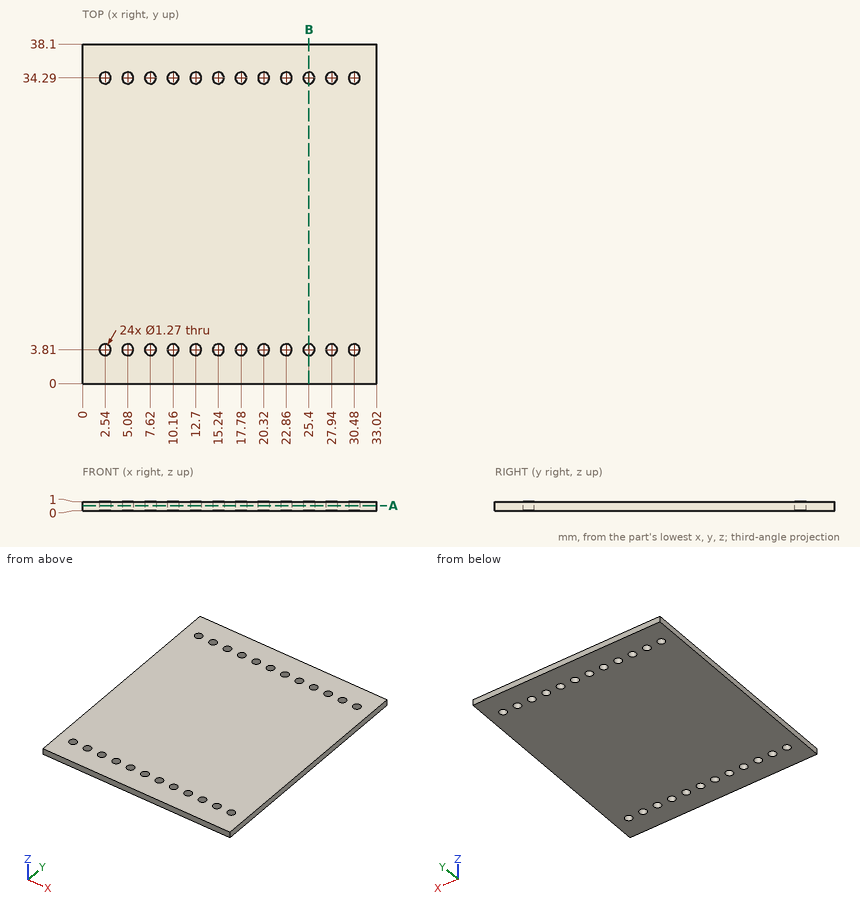
Could you check a few things on this drawing? It's one solid part, dimensions in mm from its lowest x, y, z. Give positions to 0.01 mm unless a question says otherwise; leave off trailing zeros. Order: outer loops, then holes, each group sorted by start corner. A loop starts at its lowest first (then second) coordinate and runs counter-clockwise, first axis right, second up. Notation, with made-up numbers: (-40, 72) -> (-29, 72) arc R22 ccw to (-29, 84) -> close; hole circle Ø1 at (44, 84). An arc over 180 degrees is marked (long way). Use CSV: the item, a comma, the result in double quotes. Start each with the question number.
Item 1: Suppose I cut it at B-B (x = 25.4). List the corners of the cut face in (y, z) for me (3 decimals).
Item 2: Suppose I cut it at A-A (z = 0.55). Give the number of separate pieces and of enclosed holes in the cut face, and give its area (3 significant figures).
Item 3: I'm going to push a flat-ended pin straight in: P1, Ø1, axis at x = 5.08, y = 3.81, coming from the -Z side. Where does the tip first touch, or does it pass through?
Item 4: If I drill on probe 1 along Y at (x, z) = (22.86, 0.2) (3 decimals); probe 2 along Y at (x, z) = (3, 0.7), over which ranges is the centre line in solid material (lowest first)? Write a range as [from, to].
Answer block:
1,outline,"(0, 0) -> (3.175, 0) -> (3.175, 1) -> (0, 1) -> close; (4.445, 0) -> (33.655, 0) -> (33.655, 1) -> (4.445, 1) -> close; (34.925, 0) -> (38.1, 0) -> (38.1, 1) -> (34.925, 1) -> close"
2,separate pieces,"1"
2,enclosed holes,"24"
2,area,"1,230 mm^2"
3,P1,"passes through"
4,probe 1,"y = [0, 3.175], [4.445, 33.655], [34.925, 38.1]"
4,probe 2,"y = [0, 3.37], [4.25, 33.85], [34.73, 38.1]"
